from build123d import *

# Parameters (mm, degrees)
SKETCH1_W           = 143.51
SKETCH1_H           = 143.51
BOSS_EXTRUDE1_DEPTH = 5.08
CUT_EXTRUDE1_DEPTH  = 6.08
CIRPATTERN1_COUNT   = 8


with BuildPart() as part:
    # Sketch1 → Boss-Extrude1 (new body)
    with BuildSketch(Plane(origin=(0, 0, 0), x_dir=(1, 0, 0), z_dir=(0, 1, 0))):
        with Locations((71.755, 71.755)):
            Rectangle(SKETCH1_W, SKETCH1_H)
    extrude(amount=BOSS_EXTRUDE1_DEPTH)

    # Sketch3 → Cut-Extrude1 (cut, through all)
    with BuildSketch(Plane(origin=(0, 5.08, 0), x_dir=(1, 0, 0), z_dir=(0, 1, 0))):
        with BuildLine():
            Line((71.755, 128.905), (71.755, 123.825))
            ThreePointArc((71.755, 123.825), (81.913353067, 122.824489551), (91.681326323, 119.861407258))
            Line((91.681326323, 119.861407258), (93.62535816, 124.554715283))
            ThreePointArc((93.62535816, 124.554715283), (82.904411903, 127.806878775), (71.755, 128.905))
        make_face()
    cut_extrude1 = extrude(amount=-CUT_EXTRUDE1_DEPTH, mode=Mode.SUBTRACT)

    # CirPattern1: Cut-Extrude1 ×8 about axis
    cirpattern1_axis = Axis((71.698667162, 0, -71.471795698), (0, 1, 0))
    for i in range(1, CIRPATTERN1_COUNT):
        add(cut_extrude1.rotate(cirpattern1_axis, i * 360 / CIRPATTERN1_COUNT), mode=Mode.SUBTRACT)


solid = part.part
Source: CAD feature listing. Evaluate the final solid. Frame: model axes, mm. A direction names the side the tool comes from. Round coordinates to 2 decimals unless told otherwise and drop trailing zeros. Loops run counter-clockwise (first coordinate to the right, second up) from the corner with the lowest first, then second, coordinate; pieces in that order, holes last. Notation, with made-up numbers: (82.5, -16) -> (136.5, -16) arc R24 ccw to (136.5, 21) -> close; hole circle Ø9 at (57.5, 43). An arc over 180 degrees is marked (long way). Answer as a JSON object with one key per item and string values. Group by question number.
Q1. Ray query, line 1 (Z direction, x = 110, y = 0.8); line 2 (X direction, y = 4, z = -34); line 3 (Z direction, x = 71.5, y = 3.5). Return the intervals inside material, ascending. Write a range as from..to.
Q2. Section query B-B (z = -65.5). Output: boundary loops of the cut face in (x, y), plus the area to 3 significant figures.
Q3. Section query C-C (y = 2.6). State how many separate pieces and enclosed holes the cut face has, plus the area to 3 significant figures.
Q4. Section query A-A (x = 87). Output: boundary loops of the cut face in (y, z).
Q5. Access query for faces 5 (the flat face through (50.654, 2.576, -122.132)), 6 (the flat face through (71, 0, -73)). Directions: +Z, -Z, +X, -X, +Y, -Y. A direction counts if a zero-diameter tool reaches every point of the face in a straight line with its end or side. Return the directions, or none.
Q6. Mould query, pull axis Z, two halves, no side actions, for faces 1 (the flat face through (71, 3, 0)), 2 (the flat face through (92.744, 2.576, -20.811)), 3 (the cylindrical face through (103.479, 2.576, -23.626)), 4 (the flat face through (0, 3, -71)). Classes: pulls with the +Z half, pulls with the -Z half, needs draft (parallel to the pull), parting line crosses it, or undercut.
Completed:
{
 "1": {"line 1": "-143.51..-109.69, -107.17..-33.09, -28.67..0", "line 2": "0..28.17, 34.15..108.26, 109.09..143.51", "line 3": "-143.51..-19.12, -14.04..0"},
 "2": {"outline": "(0, 0) -> (123.71, 0) -> (123.71, 5.08) -> (0, 5.08) -> close; (128.82, 0) -> (143.51, 0) -> (143.51, 5.08) -> (128.82, 5.08) -> close", "area": "703 mm²"},
 "3": {"separate pieces": "1", "enclosed holes": "8", "area": "19,700 mm²"},
 "4": {"outline": "(0, -143.51) -> (5.08, -143.51) -> (5.08, -126.83) -> (0, -126.83) -> close; (0, -121.54) -> (5.08, -121.54) -> (5.08, 0) -> (0, 0) -> close"},
 "5": {"face 5": "+Y, -Y", "face 6": "+Z, -Z, +X, -X, -Y"},
 "6": {"face 1": "pulls with the +Z half", "face 2": "undercut", "face 3": "undercut", "face 4": "needs draft"}
}
